```python
from build123d import *

# Parameters (mm, degrees)
SKETCH1_R           = 165.1
BOSS_EXTRUDE1_DEPTH = 3
SKETCH2_R           = 7.62
CUT_EXTRUDE1_DEPTH  = 2.032


with BuildPart() as part:
    # Sketch1 → Boss-Extrude1 (new body)
    with BuildSketch(Plane(origin=(0, 0, 0), x_dir=(1, 0, 0), z_dir=(0, 1, 0))):
        Circle(SKETCH1_R)
    extrude(amount=BOSS_EXTRUDE1_DEPTH)

    # Sketch2 → Cut-Extrude1 (cut)
    with BuildSketch(Plane(origin=(0, 3, 0), x_dir=(1, 0, 0), z_dir=(0, 1, 0))):
        with Locations((0, 137.4902)):
            Circle(SKETCH2_R)
        with Locations((119.070005971, -68.7451)):
            Circle(SKETCH2_R)
        with Locations((-119.070005971, -68.7451)):
            Circle(SKETCH2_R)
    extrude(amount=-CUT_EXTRUDE1_DEPTH, mode=Mode.SUBTRACT)


solid = part.part
```
Source: CAD feature listing. Evaluate the final solid. Frame: model axes, mm. A direction names the side the tool comes from. Coordinates: 2 decimals unless noted, no trailing zeros. Write each loop counter-clockwise with the first axis right and the second up, starting at its lowest first coordinate (ties: lowest second). Pieces come first, ordered by that corner, then holes. Notation, with made-up numbers: (26.5, 71) -> (61.5, 71) arc R19 ccw to (61.5, 106) -> close; hole circle Ø3 at (51.5, -23). An arc over 180 degrees is marked (long way). Return JSON: item names as keys, results as strings. Group by question number.
1) Section query C-C, the plane z = -72. Return loops of the section in (x, y), plus the area to 3 significant figures.
2) Ray query, line 1 along Z through (x, y) = (-113.5, 1.2); line 2 along X through (y, z) = (2.8, 101.5); line 3 along Z through (x, y) = (55.5, 2.35). Return the intervals inside material, ascending.
3) Mould query, pull axis Z, two halves, no side actions, for faces 1 (the face through (-35.79, 1.479, 161.174)), 2 (the face through (119, 0.968, 69)), 3 (the face through (-2, 0, -2)). Classes: +Z half, -Z half, draft (parallel to the pull), parting line (faces both ways), or undercut.
4) Contact query for flat-ended pins moving along their axis: P1, Ø1.5, axis at x = 59.5, y = 2, coming from the +Z side; P2, Ø1.5, axis at x = 17.5, y = 2, coming from the -Z side; P3, Ø1, axis at y = 0.5, z = -79.5, coming from the -X side. Output: stop coordinate, or through.
5) Section query B-B, the plane y = 0.45. Return loops of the section in (x, z), plus the area to 3 significant figures.
6) Set-up query: faces 4 (the face through (-119, 0.968, 69)), 5 (the face through (-2, 3, -2)). Return all of +Z, -Z, +X, -X, +Y, -Y with unobstructed straight access to the full face (end or side cutting, diameter ignored); none if empty.
7) Section query A-A, the plane x = 0. Return loops of the section in (y, z).
8) Section query D-D, the plane x = 90. Return loops of the section in (y, z).
From the geometry:
{
 "1": {"outline": "(-148.57, 0) -> (148.57, 0) -> (148.57, 3) -> (-148.57, 3) -> close", "area": "891 mm²"},
 "2": {"line 1": "-119.9 to 63.55, 73.95 to 119.9", "line 2": "-130.21 to 130.21", "line 3": "-155.49 to 155.49"},
 "3": {"face 1": "parting line", "face 2": "undercut", "face 3": "draft"},
 "4": {"P1": "z = 154.29", "P2": "z = -164.25", "P3": "x = -144.97"},
 "5": {"outline": "circle Ø330.2 at (0, 0)", "area": "85,600 mm²"},
 "6": {"face 4": "+Y", "face 5": "+Z, -Z, +X, -X, +Y"},
 "7": {"outline": "(0, -165.1) -> (3, -165.1) -> (3, -145.11) -> (0.97, -145.11) -> (0.97, -129.87) -> (3, -129.87) -> (3, 165.1) -> (0, 165.1) -> close"},
 "8": {"outline": "(0, -138.41) -> (3, -138.41) -> (3, 138.41) -> (0, 138.41) -> close"}
}
